Part model, mm, in its own coordinate system. Round coordinates to 2 decimals unless told otherwise and drop trailing zeros.
1) Mould opens along Z. For faces 1 (the cylindrical face through (71.85, -9.86, 52.28)), 2 (the flat face through (31, 0, 3)), 3 (the cylindrical face through (-124.88, -12.66, -5.5)) say: +Z half, -Z half, draft (parallel to the pull), parting line (faces both ways), or undercut.
2) Probe line 1 (X direction, y = -6, z = 0) (3 decimals); line 2 (X direction, y = -18, z = -3); line 3 (X direction, y = -9, z = 58). List the from-to ranges inside material, lowest first.
3) Drop flat-ended pins along their axis: P1, Ø8, axis at y = -25.5, z = -27, coming from the +X side; P2, Ø6, axis at x = 54.5, z = -47.5, coming from the -Y side; P3, Ø1, axis at x = -39, y = -16, coming from the +Z side. Give the stop position or say it passes through.
4) Band-saw the part on A-A, the plane y = -17. State how many separate pieces and enclosed holes the cut face has, then the cut area to 3 significant figures.
from build123d import *

# Parameters (mm, degrees)
CUT_EXTRUDE_THIN1_DEPTH      = 15
CUT_EXTRUDE_THIN1_DEPTH_BACK = 20


with BuildPart() as part:
    # Sketch1 → Base-Revolve (revolve)
    with BuildSketch(Plane.XY):
        with BuildLine():
            Line((19.05, 5), (24, 5))
            Line((24, 5), (25, 4))
            Line((25, 4), (25, 1))
            ThreePointArc((25, 1), (25.292893219, 0.292893219), (26, 0))
            Line((26, 0), (124, 0))
            Line((124, 0), (125, -1))
            Line((125, -1), (125, -24))
            Line((125, -24), (124, -25))
            Line((124, -25), (26, -25))
            ThreePointArc((26, -25), (25.292893219, -25.292893219), (25, -26))
            Line((25, -26), (25, -29))
            Line((25, -29), (24, -30))
            Line((24, -30), (19.05, -30))
            Line((19.05, -30), (19.05, 5))
        make_face()
    revolve(axis=Axis((0, -30350, 0), (0, 1, 0)))

    # Sketch2 → Cut-Extrude-Thin1 (cut, two sides)
    with BuildSketch(Plane(origin=(0, 0, 0), x_dir=(1, 0, 0), z_dir=(0, 1, 0))) as cut_extrude_thin1_sk:
        with BuildLine():
            ThreePointArc((109.524986247, -0.054887133), (109.229921991, 7.423375501), (108.184717895, 14.834112532))
            ThreePointArc((108.184717895, 14.834112532), (106.043659804, 22.548927161), (102.756924095, 29.84960267))
            ThreePointArc((102.756924095, 29.84960267), (98.332860497, 36.567183371), (92.916011248, 42.513272287))
            ThreePointArc((92.916011248, 42.513272287), (87.141221214, 47.295885443), (80.843977188, 51.366058191))
            ThreePointArc((80.843977188, 51.366058191), (75.279655517, 54.316272842), (69.579158541, 56.993916655))
            ThreePointArc((69.579158541, 56.993916655), (65.230785476, 58.999236045), (60.953055197, 61.151137028))
            ThreePointArc((60.953055197, 61.151137028), (57.290135984, 63.276226982), (53.749285638, 65.599019115))
            ThreePointArc((53.749285638, 65.599019115), (49.601954473, 68.481518372), (45.406369026, 71.293318599))
            ThreePointArc((45.406369026, 71.293318599), (-71.312570217, 45.376127579), (-45.345877971, -71.331809006))
            ThreePointArc((-45.345877971, -71.331809006), (-38.593898018, -75.405527827), (-31.649923168, -79.142589722))
            ThreePointArc((-31.649923168, -79.142589722), (-24.034421899, -82.711545409), (-16.211151125, -85.798572893))
            ThreePointArc((-16.211151125, -85.798572893), (-7.620932162, -88.510877367), (1.153325471, -90.550696085))
            ThreePointArc((1.153325471, -90.550696085), (10.620649637, -91.921398106), (20.173660561, -92.420430343))
            ThreePointArc((20.173660561, -92.420430343), (30.195991067, -91.960061817), (40.115734041, -90.457481608))
            ThreePointArc((40.115734041, -90.457481608), (50.164053761, -87.778443627), (59.835395829, -83.955994636))
            ThreePointArc((59.835395829, -83.955994636), (69.217053614, -78.865285844), (77.888616734, -72.641556104))
            ThreePointArc((77.888616734, -72.641556104), (85.826699629, -65.22323814), (92.717665183, -56.823286045))
            ThreePointArc((92.717665183, -56.823286045), (98.476591418, -47.488521124), (102.919592608, -37.460420212))
            ThreePointArc((102.919592608, -37.460420212), (107.856238797, -19.046190631), (109.524986247, -0.054887133))
        make_face()
        with BuildLine():
            ThreePointArc((90.474982456, 0.056342792), (90.262741838, 5.647173284), (89.486847533, 11.187969228))
            ThreePointArc((89.486847533, 11.187969228), (88.12991005, 16.068178084), (86.054133631, 20.688661832))
            ThreePointArc((86.054133631, 20.688661832), (83.284958022, 24.885433828), (79.899946609, 28.603353472))
            ThreePointArc((79.899946609, 28.603353472), (75.875178075, 31.93428485), (71.488414915, 34.771567807))
            ThreePointArc((71.488414915, 34.771567807), (66.751022738, 37.282035549), (61.898062734, 39.56109503))
            ThreePointArc((61.898062734, 39.56109503), (56.897401317, 41.868517981), (51.979131099, 44.346709525))
            ThreePointArc((51.979131099, 44.346709525), (47.310945971, 47.049113929), (42.801511531, 50.008834013))
            ThreePointArc((42.801511531, 50.008834013), (38.952515201, 52.685804726), (35.059073926, 55.297712072))
            ThreePointArc((35.059073926, 55.297712072), (-55.279422123, 35.087905534), (-35.1167276, -55.261117141))
            ThreePointArc((-35.1167276, -55.261117141), (-29.160317457, -58.855298852), (-23.034341253, -62.152173057))
            ThreePointArc((-23.034341253, -62.152173057), (-16.494338073, -65.217270915), (-9.775872963, -67.868439157))
            ThreePointArc((-9.775872963, -67.868439157), (-2.592647115, -70.136469906), (4.744453336, -71.842240708))
            ThreePointArc((4.744453336, -71.842240708), (12.484550044, -72.962801762), (20.294689574, -73.370814789))
            ThreePointArc((20.294689574, -73.370814789), (28.32982468, -73.001688389), (36.282721862, -71.797081864))
            ThreePointArc((36.282721862, -71.797081864), (44.198795786, -69.686506265), (51.817937068, -66.675286938))
            ThreePointArc((51.817937068, -66.675286938), (59.100153222, -62.723698973), (65.831324035, -57.892854425))
            ThreePointArc((65.831324035, -57.892854425), (71.928664779, -52.194534162), (77.221947559, -45.742435637))
            ThreePointArc((77.221947559, -45.742435637), (81.623193338, -38.607897611), (85.018936267, -30.943595477))
            ThreePointArc((85.018936267, -30.943595477), (89.105431486, -15.682719937), (90.474982456, 0.056342792))
        make_face(mode=Mode.SUBTRACT)
    extrude(amount=CUT_EXTRUDE_THIN1_DEPTH, mode=Mode.SUBTRACT)
    extrude(cut_extrude_thin1_sk.sketch, amount=-CUT_EXTRUDE_THIN1_DEPTH_BACK, mode=Mode.SUBTRACT)


solid = part.part
Reported:
1. face 1: undercut
1. face 2: draft
1. face 3: parting line
2. line 1: x = -125 to -84.525, -65.475 to -19.05, 19.05 to 90.475, 109.526 to 125
2. line 2: x = -124.96 to -84.47, -65.41 to -18.81, 18.81 to 90.43, 109.5 to 124.96
2. line 3: x = -110.73 to -61.49, -30.64 to 65.7, 91.86 to 110.73
3. P1: stops at x = 122.81
3. P2: stops at y = -25
3. P3: stops at z = 118.92
4. separate pieces: 2
4. enclosed holes: 2
4. area: 38,000 mm2
